Autodesk Inventor part; units mm, degrees
ref_plane "YZ Plane" through (0, 0, 0) normal (1, 0, 0) x (0, 1, 0)
ref_plane "XZ Plane" through (0, 0, 0) normal (0, 1, 0) x (-1, 0, 0)
ref_plane "XY Plane" through (0, 0, 0) normal (0, 0, 1) x (1, 0, 0)
sketch "Sketch1" plane through (0, 0, 0) normal (0, 0, 1) x (1, 0, 0)
  line L0 (-25, -32.5) -> (25, -32.5)
  line L1 (25, -32.5) -> (25, 32.5)
  line L2 (25, 32.5) -> (-25, 32.5)
  line L3 (-25, 32.5) -> (-25, -32.5)
  line L4 (-25, -32.5) -> (25, 32.5) construction
  line L5 (25, -32.5) -> (-25, 32.5) construction
  circle A0 centre (0, 17.5) radius 6.85
  point P0 (0, 0)
  dimension "d0" = 50
  dimension "d1" = 13.7
  dimension "d2" = 50
  dimension "d3" = 65
extrude "Plate1" add sketch "Sketch1" along normal blind 3
sketch "Sketch2" plane through (-22, -32.5, 0) normal (-1, 0, 0) x (0, -1, 0)
  line L0 (-65, 0) -> (0, 0)
  line L1 (0, 0) -> (0, 45)
  line L2 (0, 45) -> (-65, 45)
  line L3 (-65, 45) -> (-65, 0)
edge flange "Flange1" height 45 angle 90 thickness 3 bend radius 3 thickness toward (-1, 0, 0) relief tear relief width 3 relief depth 1.5 corner gap 3 corner form 0 edges at (-25, 0, 3) (25, 0, 3) wall of the first edge with corners at (-22, 32.5, 0) (-22, -32.5, 0) (-22, -32.5, 45) (-22, 32.5, 45)
bend "Bend1"
corner "Corner1"
sketch "Sketch3" plane through (25, -32.5, 45) normal (1, 0, 0) x (0, 0, -1)
  line L0 (0, 65) -> (0, 0)
  line L1 (0, 0) -> (40.9053, 68.1756)
  line L2 (40.9053, 68.1756) -> (0, 68.1756)
  line L3 (0, 68.1756) -> (0, 0)
  point P0 (45, 32.5)
  point P1 (0, 65)
  point P2 (39, 65)
extrude "Extrusion1" cut sketch "Sketch3" against normal through all
fillet "Fillet1" radius 5 2 edges at (-23.5, 32.5, 6) (23.5, 32.5, 6)
equation "\"d4\" = Thickness"
equation "\"d5\" = BendReliefWidth"
equation "\"d6\" = BendReliefDepth"
equation "\"d7\" = MinimumRemnant"
equation "\"d8\" = TransitionRadius"
equation "\"d11\" = BendRadius"
equation "\"d12\" = CornerReliefSize"
equation "\"d13\" = GapSize"
equation "\"d14\" = JacobiRadiusSize"
equation "\"BendRadius\" = Thickness"
equation "\"BendReliefWidth\" = Thickness"
equation "\"BendReliefDepth\" = 0.5 * Thickness"
equation "\"CornerReliefSize\" = 4 * Thickness"
equation "\"MinimumRemnant\" = 2 * Thickness"
equation "\"TransitionRadius\" = BendRadius"
equation "\"JacobiRadiusSize\" = BendRadius"
equation "\"GapSize\" = Thickness"
properties part number "Soporte Fijo"
Here's how the part is built. I have some questions about the finished solid (model axes, mm). A direction names the side the tool comes from. Round coordinates to 2 decimals unless told otherwise and drop trailing zeros. Order: outer loops, then holes, each group sorted by start corner. A loop starts at its lowest first (then second) coordinate and runs counter-clockwise, first axis right, second up. Notation, with made-up numbers: M 42.5,-35 L 64.5,-35 A5 cw 64.5,-30 Z; hole C 8.5,66.25 d5. An arc over 180 degrees is marked long. Answer in a Markdown table with one row per item.
Item 1: Imagine slicing it at D-D, the plane y = -26. Write out the boundary of the cut face in (x, z).
A:
| item | result |
|---|---|
| outline | M -25,6 A6 ccw -19,0 L 19,0 A6 ccw 25,6 L 25,41.1 L 22,41.1 L 22,6 A3 cw 19,3 L -19,3 A3 cw -22,6 L -22,41.1 L -25,41.1 Z |
Item 2: I'm going to push a flat-ended pin straight in: pin 1 (3 mm diameter, centred on x = -4.5, y = -8.5, fed in from +Z). Where does the tip first touch, or does it pass through?
A:
| item | result |
|---|---|
| pin 1 | stops at z = 3 |
Item 3: For faces 4 (the face through (23.52, -1.65, 26.49)), 5 (the face through (-21.14, -0.45, 3.9)), which set-ups out of +Z, -Z, +X, -X, +Y, -Y let a thin tool reach every point of the face, with its end or its side?
A:
| item | result |
|---|---|
| face 4 | +Z, +X, -X, +Y |
| face 5 | +Z, +Y, -Y |
Item 4: If I drill on L1, parallel to Y at x = 0, z = 1; L2, parallel to X at y = -21, z = 29; L3, parallel to Z at x = 9, y = 21, over which ranges is the centre line in solid material (lowest first)? Write a range as from..to.
A:
| item | result |
|---|---|
| L1 | y = -32.5..10.65, 24.35..32.5 |
| L2 | x = -25..-22, 22..25 |
| L3 | z = 0..3 |
Item 5: Thinking about a two-plate mould opening in X: for faces 1 (the face through (23.289, 0.455, 1.804)), 2 (the face through (0, 0, 0)), 3 (the face through (21.14, 0.45, 3.9)), which applies, +X half, -X half, draft (parallel to the pull), parting line (faces both ways), or undercut?
A:
| item | result |
|---|---|
| face 1 | +X half |
| face 2 | draft |
| face 3 | undercut |
Item 6: Imagine slicing it at C-C, the plane y = 17.5. Write out the boundary of the cut face in (x, z).
A:
| item | result |
|---|---|
| outline | M -25,6 A6 ccw -19,0 L -6.85,0 L -6.85,3 L -19,3 A3 cw -22,6 L -22,15 L -25,15 Z; M 6.85,0 L 19,0 A6 ccw 25,6 L 25,15 L 22,15 L 22,6 A3 cw 19,3 L 6.85,3 Z |
Item 7: Imagine slicing it at A-A, the plane x = 0. Write out the boundary of the cut face in (y, z).
A:
| item | result |
|---|---|
| outline | M -32.5,0 L 10.65,0 L 10.65,3 L -32.5,3 Z; M 24.35,0 L 32.5,0 L 32.5,3 L 24.35,3 Z |
Item 8: Imagine slicing it at B-B, the plane z = 5. Write out the boundary of the cut face in (x, y), and give its area (3 significant figures).
A:
| item | result |
|---|---|
| outline | M -24.92,-32.5 L -21.83,-32.5 L -21.83,32.15 L -24.92,32.15 Z; M 21.83,-32.5 L 24.92,-32.5 L 24.92,32.15 L 21.83,32.15 Z |
| area | 399 mm2 |
